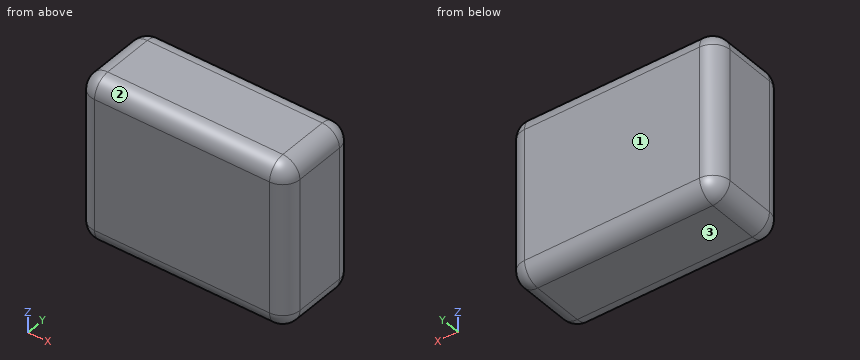
from build123d import *

# Parameters (mm, degrees)
F0_W     = 93.1164
F0_H     = 73.66
F1_DEPTH = 19.05
F2_R     = 7.62
F3_R     = 7.62
F4_R     = 7.62


with BuildPart() as f1:
    # F0 (on Front) → F1 (new body, symmetric)
    with BuildSketch(Plane.XZ):
        Rectangle(F0_W, F0_H)
    extrude(amount=F1_DEPTH, both=True)

    # F2
    f2_edges = [f1.edges().sort_by_distance(p)[0] for p in [
        (-46.5582, 0, -36.83),
        (-46.5582, 0, 36.83),
        (46.5582, 0, -36.83),
        (46.5582, 0, 36.83),
    ]]
    fillet(f2_edges, radius=F2_R)

    # F3
    f3_edges = [f1.edges().sort_by_distance(p)[0] for p in [
        (44.326354, -19.05, -34.598154),
        (0, -19.05, -36.83),
        (46.5582, -19.05, 0),
        (44.326354, -19.05, 34.598154),
        (0, -19.05, 36.83),
        (-44.326354, -19.05, 34.598154),
        (-46.5582, -19.05, 0),
        (-44.326354, -19.05, -34.598154),
    ]]
    fillet(f3_edges, radius=F3_R)

    # F4
    f4_edges = [f1.edges().sort_by_distance(p)[0] for p in [
        (44.326354, 19.05, -34.598154),
        (0, 19.05, -36.83),
        (46.5582, 19.05, 0),
        (-44.326354, 19.05, -34.598154),
        (-46.5582, 19.05, 0),
        (-44.326354, 19.05, 34.598154),
        (0, 19.05, 36.83),
        (44.326354, 19.05, 34.598154),
    ]]
    fillet(f4_edges, radius=F4_R)


solid = f1.part
Geometry check sheet. Reference: the model listing, model coordinates, mm. Face numbers are marked on the shaded views. Give positions to 0.01 mm unless a question says otherwise; leave off trailing zeros. Loops run counter-clockwise (first coordinate to the right, second up) from the corner with the lowest first, then second, coordinate; pieces in that order, holes last. Notation, with made-up numbers: M 32,-5.75 L 90,-5.75 A20 ccw 90,9.25 Z; hole C 71,-19.75 d9. An arc over 180 degrees is marked long. Answer as a JSON object with one key per item and string values. Group by question number.
Item 1: Sectioned sample at A-A on x = -33.5. Record the boundary of the cut face in (y, z).
Item 2: Sectioned sample at B-B on z = 31.5. Record the boundary of the cut face in (x, y), plus the area to 3 significant figures.
Item 3: Material ranges on L1, parallel to Z at x = -39.5, y = 10; L2, parallel to X at y = 11.5, z = 18.5; L3, parallel to X at y = -12, z = -15, recorded low to high.
Item 4: Mould release check, pull along Y, two halves, no side actions. Record for the marked faces 1, 2 and 3: pulls with the +Y half, pulls with the -Y half, needs draft (parallel to the pull), parting line crosses it, or undercut.
Findings below:
{
 "1": {"outline": "M -19.05,-29.21 A7.62 ccw -11.43,-36.83 L 11.43,-36.83 A7.62 ccw 19.05,-29.21 L 19.05,29.21 A7.62 ccw 11.43,36.83 L -11.43,36.83 A7.62 ccw -19.05,29.21 Z"},
 "2": {"outline": "M -46.21,-11.43 A7.27 ccw -38.94,-18.7 L 38.94,-18.7 A7.27 ccw 46.21,-11.43 L 46.21,11.43 A7.27 ccw 38.94,18.7 L -38.94,18.7 A7.27 ccw -46.21,11.43 Z", "area": "3,410 mm2"},
 "3": {"L1": "-36.81 to 36.81", "L2": "-46.56 to 46.56", "L3": "-46.54 to 46.54"},
 "4": {"face 1": "pulls with the +Y half", "face 2": "pulls with the -Y half", "face 3": "needs draft"}
}
